Build history of the part. All positions in model axes, mm. Round coordinates to 2 decimals unless told otherwise and drop trailing zeros. Write each loop counter-clockwise with the first axis right and the second up, starting at its lowest first coordinate (ties: lowest second). Pieces come first, ordered by that corner, then holes. Notation, with made-up numbers: (-26.5, -24.5) - (-18.5, -24.5) arc R21 cw to (-18.5, -15.5) - close; hole circle Ø7 at (36.25, 69). An arc over 180 degrees is marked (long way). Answer as a JSON object with one key per item and string values. Group by question number.
Item 1: Flat gauge pins, fed straight in: pin 1 (1 mm diameter, centred on x = 3, z = 75.5, fed in from -Y); pin 2 (1 mm diameter, centred on y = -0.5, z = 73, fed in from +X); pin 3 (5 mm diameter, centred on x = -3, z = 85, fed in from -Y). Where does each tip first touch, or does it go through?
Item 2: Slice it at B-B, the plane y = 0. List the corners of the cut face in (x, z).
Item 3: Slice it at D-D, the plane z = 74.5. List the corners of the cut face in (x, y), then the cut area to 3 significant figures.
Item 4: Slice it at C-C, the plane x = 0. List the corners of the cut face in (y, z), then the cut area to 3 significant figures.
Item 5: Slice it at A-A, the plane z = 0. List the corners of the cut face in (x, y), then the cut area to 3 significant figures.
Item 6: Probe line 1 (Y direction, x = -2, z = 0); line 2 (Z direction, x = -0.75, y = 1); line 3 (X direction, y = 0, z = 35.5). List the from-to ranges inside material, lowest first. Write a range as from..to.
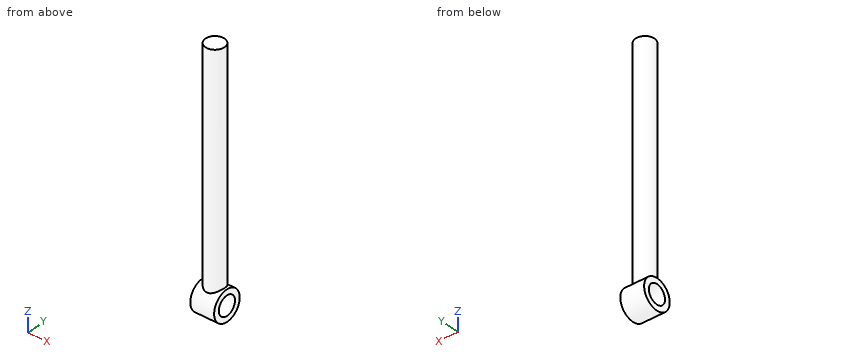
from build123d import *

# Parameters (mm, degrees)
SKETCH2_R           = 4
BOSS_EXTRUDE1_DEPTH = 100
SKETCH1_R           = 6.35
BOSS_EXTRUDE2_DEPTH = 5.08
SKETCH1_3_R         = 4
CUT_EXTRUDE1_DEPTH  = 5.08


with BuildPart() as part:
    # Sketch2 → Boss-Extrude1 (new body)
    with BuildSketch(Plane(origin=(0, 0, 0), x_dir=(0, 1, 0), z_dir=(0, 0, 1))):
        with Locations(Location((0, 0, 0), (0, 0, 270))):
            Circle(SKETCH2_R)
    extrude(amount=BOSS_EXTRUDE1_DEPTH)

    # Sketch1 → Boss-Extrude2 (add, symmetric)
    with BuildSketch(Plane.YZ):
        with Locations(Location((0, 0, 0), (0, 0, 270))):
            Circle(SKETCH1_R)
    extrude(amount=BOSS_EXTRUDE2_DEPTH, both=True)

    # Sketch1_3 → Cut-Extrude1 (cut, symmetric)
    with BuildSketch(Plane.YZ):
        with Locations(Location((0, 0, 0), (0, 0, 270))):
            Circle(SKETCH1_3_R)
    extrude(amount=CUT_EXTRUDE1_DEPTH, both=True, mode=Mode.SUBTRACT)


solid = part.part
Geometry says:
{
 "1": {"pin 1": "stops at y = -3.12", "pin 2": "stops at x = 4", "pin 3": "stops at y = -3.97"},
 "2": {"outline": "(-5.08, -6.35) - (5.08, -6.35) - (5.08, -4) - (-5.08, -4) - close; (-5.08, 4) - (5.08, 4) - (5.08, 6.35) - (4, 6.35) - (4, 100) - (-4, 100) - (-4, 6.35) - (-5.08, 6.35) - close"},
 "3": {"outline": "circle Ø8 at (0, 0)", "area": "50.3 mm^2"},
 "4": {"outline": "(-4, 4.93) arc R6.35 ccw (long way) to (4, 4.93) - (4, 100) - (-4, 100) - close; hole circle Ø8 at (0, 0)", "area": "829 mm^2"},
 "5": {"outline": "(-5.08, -6.35) - (5.08, -6.35) - (5.08, -4) - (-5.08, -4) - close; (-5.08, 4) - (5.08, 4) - (5.08, 6.35) - (-5.08, 6.35) - close", "area": "47.8 mm^2"},
 "6": {"line 1": "y = -6.35..-4, 4..6.35", "line 2": "z = -6.27..-3.87, 3.87..100", "line 3": "x = -4..4"}
}
